Geometry: final body of the model. Coordinates: model frame, mm. Give positions to 0.01 mm unless a question says otherwise; leave off trailing zeros. Write each loop counter-clockwise with the first axis right and the second up, starting at its lowest first coordinate (ties: lowest second). Pieces come first, ordered by that corner, then holes. Notation, with made-up numbers: (30, 84) -> (81, 84) arc R17 ccw to (81, 99) -> close; hole circle Ø10 at (20, -6.5). An arc over 180 degrees is marked (long way). Use CSV: the item, a comma, the result in double quotes. Start each with the question number.
1) Section A-A (y = 4). Count the separate pieces of the cut face and the enclosed holes in it, plus the area to 3 significant figures.
2) Section D-D (x = -36). Output: boundary loops of the cut face in (y, z).
3) Contact query for flat-ended pins moving along their axis: P1, Ø3, axis at x = -25, y = 5, coming from the +Z side; P2, Ø1.1, axis at y = 0.5, z = -45, coming from the -X side; P3, Ø10, axis at x = -31.5, z = 6.5, coming from the +Y side. Output: stop coordinate, or through.
4) Section C-C (z = 24.5). Output: boundary loops of the cut face in (x, y), plus the area to 3 significant figures.
5) Material intervals for line 1 (Z direction, x = 10, y = 1.75); line 2 (X direction, y = 1.5, z = 5.5); line 3 (Y direction, x = -31, z = 8), sorted ascending. Write a range as [from, to].
6) Section B-B (x = 25.5). Output: boundary loops of the cut face in (y, z).
```python
from build123d import *

# Parameters (mm, degrees)
SKETCH1_W           = 0.2
SKETCH1_H           = 2.5
SKETCH1_W_2         = 82.6
SKETCH1_H_2         = 100
BOSS_EXTRUDE1_DEPTH = 2.23
SKETCH2_W           = 7.4
SKETCH2_H           = 3.75
SKETCH2_H_2         = 3
BOSS_EXTRUDE2_DEPTH = 4
SKETCH3_W           = 60
SKETCH3_H           = 70
CUT_EXTRUDE1_DEPTH  = 10
CUT_EXTRUDE2_DEPTH  = 0.5
SKETCH5_W           = 7.4
SKETCH5_H           = 2
BOSS_EXTRUDE3_DEPTH = 3


with BuildPart() as part:
    # Sketch1 → Boss-Extrude1 (new body)
    with BuildSketch(Plane(origin=(0, 0, 0), x_dir=(1, 0, 0), z_dir=(0, 1, 0))):
        with BuildLine():
            Line((43.1, -36.85), (43.1, -37.5))
            ThreePointArc((43.1, -37.5), (44.922195524, -37.020142239), (46.5, -35.99))
            Line((46.5, -35.99), (46.5, -34.49))
            Line((46.5, -34.49), (43.1, -34.49))
            Line((43.1, -34.49), (43.1, -36.85))
        make_face()
        Polygon((41.5, -34.49), (41.3, -34.49), (41.3, -36.85), (43.1, -36.85), (43.1, -34.49), align=None)
        Polygon((45, -29.49), (41.3, -29.49), (41.3, -31.99), (41.5, -31.99), (46.5, -31.99), (46.5, -30.49), align=None)
        with Locations((41.4, -33.24)):
            Rectangle(SKETCH1_W, SKETCH1_H)
        Rectangle(SKETCH1_W_2, SKETCH1_H_2)
        Polygon((46.5, 43.01), (41.5, 43.01), (41.3, 43.01), (41.3, 40.51), (45, 40.51), (46.5, 41.51), align=None)
        with Locations((41.4, 44.26)):
            Rectangle(SKETCH1_W, SKETCH1_H)
        Polygon((41.5, 45.51), (43.1, 45.51), (43.1, 47.87), (41.3, 47.87), (41.3, 45.51), align=None)
        with BuildLine():
            ThreePointArc((43.1, 48.52), (44.922195524, 48.040142239), (46.5, 47.01))
            Line((46.5, 47.01), (46.5, 45.51))
            Line((46.5, 45.51), (43.1, 45.51))
            Line((43.1, 45.51), (43.1, 47.87))
            Line((43.1, 47.87), (43.1, 48.52))
        make_face()
        with BuildLine():
            Line((-43.1, -46.87), (-41.3, -46.87))
            Line((-41.3, -46.87), (-41.3, -44.51))
            Line((-41.3, -44.51), (-41.5, -44.51))
            Line((-41.5, -44.51), (-46.5, -44.51))
            Line((-46.5, -44.51), (-46.5, -46.01))
            ThreePointArc((-46.5, -46.01), (-44.922195524, -47.040142239), (-43.1, -47.52))
            Line((-43.1, -47.52), (-43.1, -46.87))
        make_face()
        Polygon((-41.3, -44.51), (-41.3, -39.51), (-45, -39.51), (-46.5, -40.51), (-46.5, -42.01), (-41.5, -42.01), (-41.5, -44.51), align=None)
        Polygon((-41.3, 30.49), (-41.3, 35.49), (-41.5, 35.49), (-41.5, 32.99), (-46.5, 32.99), (-46.5, 31.49), (-45, 30.49), align=None)
        with BuildLine():
            Line((-41.3, 35.49), (-41.3, 37.85))
            Line((-41.3, 37.85), (-43.1, 37.85))
            Line((-43.1, 37.85), (-43.1, 38.5))
            ThreePointArc((-43.1, 38.5), (-44.922195524, 38.020142239), (-46.5, 36.99))
            Line((-46.5, 36.99), (-46.5, 35.49))
            Line((-46.5, 35.49), (-41.5, 35.49))
            Line((-41.5, 35.49), (-41.3, 35.49))
        make_face()
    extrude(amount=BOSS_EXTRUDE1_DEPTH)

    # Sketch2 → Boss-Extrude2 (add)
    with BuildSketch(Plane(origin=(0, 2.23, 0), x_dir=(1, 0, 0), z_dir=(0, 1, 0))):
        with Locations((-25.2, -45.625)):
            Rectangle(SKETCH2_W, SKETCH2_H)
        with Locations((25.2, -45.625)):
            Rectangle(SKETCH2_W, SKETCH2_H)
        with Locations((25.2, 45.625)):
            Rectangle(SKETCH2_W, SKETCH2_H)
        with Locations((-25.2, 45.625)):
            Rectangle(SKETCH2_W, SKETCH2_H)
        with Locations((-25.2, 37.5)):
            Rectangle(SKETCH2_W, SKETCH2_H_2)
        with Locations((25.2, 37.5)):
            Rectangle(SKETCH2_W, SKETCH2_H_2)
    extrude(amount=BOSS_EXTRUDE2_DEPTH)

    # Sketch3 → Cut-Extrude1 (cut)
    with BuildSketch(Plane(origin=(0, 2.23, 0), x_dir=(1, 0, 0), z_dir=(0, 1, 0))):
        Rectangle(SKETCH3_W, SKETCH3_H)
    extrude(amount=-CUT_EXTRUDE1_DEPTH, mode=Mode.SUBTRACT)

    # Sketch4 → Cut-Extrude2 (cut)
    with BuildSketch(Plane.XZ):
        Polygon((4.640384615, -43.419230769), (4.640384615, -45.291666667), (4.070512821, -45.291666667), (4.070512821, -43.419230769), (2.198076923, -43.419230769), (2.198076923, -42.849358974), (4.070512821, -42.849358974), (4.070512821, -40.976923077), (4.640384615, -40.976923077), (4.640384615, -42.849358974), (6.512820513, -42.849358974), (6.512820513, -43.419230769), align=None)
        Polygon((1.221153846, -45.698717949), (1.221153846, -46.35), (-2.116666667, -46.35), (0.54697516, -40.651282051), (-2.03525641, -40.651282051), (-2.03525641, -40), (1.465384615, -40), (-1.198257212, -45.698717949), align=None)
        with BuildLine():
            add(Edge.make_bspline(
                [(-3.175, -44.482652244), (-3.262918211, -44.565594294), (-3.433284709, -44.726318068), (-3.671176807, -44.969181062), (-3.884395029, -45.204215059), (-4.071386431, -45.432230465), (-4.235563138, -45.650653984), (-4.373446797, -45.862117777), (-4.487450991, -46.065713922), (-4.546079998, -46.202765549), (-4.574238782, -46.268589744)],
                knots=[0, 0, 0, 0, 0.000362575, 0.000702591, 0.001019617, 0.001314251, 0.001586978, 0.001838892, 0.00207117, 0.002285828, 0.002285828, 0.002285828, 0.002285828], degree=3))
            Line((-4.574238782, -46.268589744), (-4.759955929, -46.268589744))
            add(Edge.make_bspline(
                [(-4.759955929, -46.268589744), (-4.792788221, -46.198486652), (-4.860615985, -46.053661673), (-4.986779978, -45.841364869), (-5.132525091, -45.623706079), (-5.300867212, -45.402881295), (-5.491310702, -45.177687257), (-5.702118152, -44.94759275), (-5.93585869, -44.714525691), (-6.101847246, -44.561381426), (-6.187179487, -44.482652244)],
                knots=[0, 0, 0, 0, 0.000232111, 0.000479514, 0.000739881, 0.001017698, 0.001312003, 0.001624408, 0.001953613, 0.002301902, 0.002301902, 0.002301902, 0.002301902], degree=3))
            Line((-6.187179487, -44.482652244), (-6.187179487, -44.151923077))
            add(Edge.make_bspline(
                [(-6.187179487, -44.151923077), (-6.116537815, -44.184471117), (-5.978890638, -44.247891839), (-5.781903944, -44.34935602), (-5.597143614, -44.448436612), (-5.427913951, -44.551377879), (-5.270864773, -44.651733434), (-5.129759329, -44.755968393), (-5.000056754, -44.857829341), (-4.922299946, -44.930706152), (-4.884615385, -44.966025641)],
                knots=[0, 0, 0, 0, 0.000233307, 0.000454604, 0.000664648, 0.000862076, 0.001048719, 0.001223511, 0.001388199, 0.001543075, 0.001543075, 0.001543075, 0.001543075], degree=3))
            Line((-4.884615385, -44.966025641), (-4.884615385, -38.127564103))
            Line((-4.884615385, -38.127564103), (-4.477564103, -38.127564103))
            Line((-4.477564103, -38.127564103), (-4.477564103, -44.966025641))
            add(Edge.make_bspline(
                [(-4.477564103, -44.966025641), (-4.378031962, -44.888388472), (-4.177950241, -44.732320508), (-3.858882125, -44.521130617), (-3.525108924, -44.32477265), (-3.292360048, -44.209864), (-3.175, -44.151923077)],
                knots=[0, 0, 0, 0, 0.000378565, 0.000760999, 0.001146938, 0.001539469, 0.001539469, 0.001539469, 0.001539469], degree=3))
            Line((-3.175, -44.151923077), (-3.175, -44.482652244))
        make_face()
    extrude(amount=-CUT_EXTRUDE2_DEPTH, mode=Mode.SUBTRACT)

    # Sketch5 → Boss-Extrude3 (add)
    with BuildSketch(Plane(origin=(0, 2.23, 0), x_dir=(1, 0, 0), z_dir=(0, 1, 0))):
        with Locations((-25.2, -40.25)):
            Rectangle(SKETCH5_W, SKETCH5_H)
        with Locations((25.2, -40.25)):
            Rectangle(SKETCH5_W, SKETCH5_H)
    extrude(amount=BOSS_EXTRUDE3_DEPTH)


solid = part.part
```
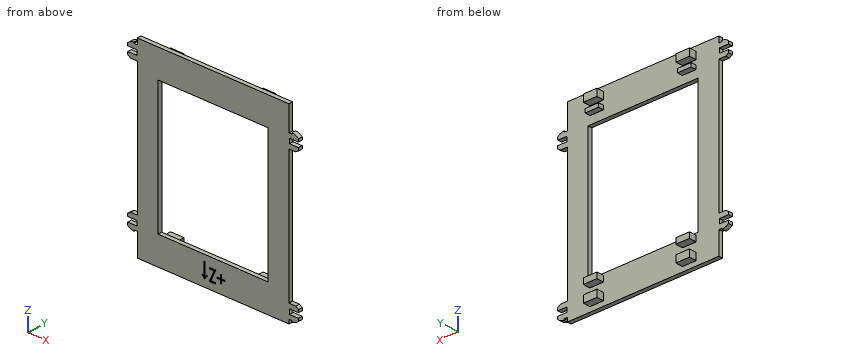
Answers follow:
1,separate pieces,"8"
1,enclosed holes,"0"
1,area,"185 mm^2"
2,outline,"(0, -50) -> (2.23, -50) -> (2.23, 50) -> (0, 50) -> close"
3,P1,"stops at z = 47.5"
3,P2,"stops at x = -41.3"
3,P3,"stops at y = 2.23"
4,outline,"(-41.3, 0) -> (-30, 0) -> (-30, 2.23) -> (-41.3, 2.23) -> close; (30, 0) -> (41.3, 0) -> (41.3, 2.23) -> (30, 2.23) -> close"
4,area,"50.4 mm^2"
5,line 1,"z = [-50, -35], [35, 50]"
5,line 2,"x = [-41.3, -30], [30, 41.3]"
5,line 3,"y = [0, 2.23]"
6,outline,"(0, -50) -> (2.23, -50) -> (2.23, -47.5) -> (6.23, -47.5) -> (6.23, -43.75) -> (2.23, -43.75) -> (2.23, -39) -> (6.23, -39) -> (6.23, -36) -> (2.23, -36) -> (2.23, -35) -> (0, -35) -> close; (0, 35) -> (2.23, 35) -> (2.23, 39.25) -> (5.23, 39.25) -> (5.23, 41.25) -> (2.23, 41.25) -> (2.23, 43.75) -> (6.23, 43.75) -> (6.23, 47.5) -> (2.23, 47.5) -> (2.23, 50) -> (0, 50) -> close"
